from build123d import *

# Parameters (mm, degrees)
BOSS_EXTRUDE1_DEPTH             = 85
BOSS_EXTRUDE1_DEPTH_BACK        = 85
BOSS_EXTRUDE2_START             = -85
SKETCH1_4_W                     = 45
SKETCH1_4_H                     = 163
BOSS_EXTRUDE2_DEPTH             = 3
BOSS_EXTRUDE3_START             = 85
SKETCH1_5_W                     = 45
SKETCH1_5_H                     = 163
BOSS_EXTRUDE3_DEPTH             = 3
BOSS_EXTRUDE4_REACH             = 192.625
BOSS_EXTRUDE4_DIRECTION_2_REACH = 192.625
SKETCH5_W                       = 10
SKETCH5_H                       = 3
BOSS_EXTRUDE7_DEPTH             = 5
BOSS_EXTRUDE8_DEPTH             = 88
BOSS_EXTRUDE8_DEPTH_BACK        = 88
CHAMFER1_SIZE                   = 5


with BuildPart() as part:
    # Sketch1 → Boss-Extrude1 (new, two sides: drawn at the far end of the back side and taken through both)
    with BuildSketch(Plane(origin=(0, 0, 0), x_dir=(0, 0, -1), z_dir=(1, 0, 0)).offset(-BOSS_EXTRUDE1_DEPTH_BACK)):
        Polygon((-45, -3), (-45, 0), (0, 0), (0, 163), (3, 163), (3, -3), align=None)
    extrude(amount=BOSS_EXTRUDE1_DEPTH + BOSS_EXTRUDE1_DEPTH_BACK)

    # Sketch1<4> → Boss-Extrude2 (add)
    with BuildSketch(Plane(origin=(0, 0, 0), x_dir=(0, 0, -1), z_dir=(1, 0, 0)).offset(BOSS_EXTRUDE2_START)):
        with Locations((-22.5, 81.5)):
            Rectangle(SKETCH1_4_W, SKETCH1_4_H)
        Polygon((-45, -3), (-45, 0), (0, 0), (0, 163), (3, 163), (3, -3), align=None)
    extrude(amount=-BOSS_EXTRUDE2_DEPTH)

    # Sketch1<5> → Boss-Extrude3 (add)
    with BuildSketch(Plane(origin=(0, 0, 0), x_dir=(0, 0, -1), z_dir=(1, 0, 0)).offset(BOSS_EXTRUDE3_START)):
        Polygon((-45, -3), (-45, 0), (0, 0), (0, 163), (3, 163), (3, -3), align=None)
        with Locations((-22.5, 81.5)):
            Rectangle(SKETCH1_5_W, SKETCH1_5_H)
    extrude(amount=BOSS_EXTRUDE3_DEPTH)

    # Sketch2 → Boss-Extrude4 (add, up to next)
    with BuildSketch(Plane(origin=(0, 0, 0), x_dir=(0, 0, -1), z_dir=(1, 0, 0)), mode=Mode.PRIVATE) as boss_extrude4_sk1:
        Polygon((-10, 160), (-10, 150), (0, 140), (0, 160), align=None)
    boss_extrude4_tool1 = extrude(boss_extrude4_sk1.sketch, amount=BOSS_EXTRUDE4_REACH, mode=Mode.PRIVATE) - part.part
    add(boss_extrude4_tool1.solids().sort_by_distance((0, 152.222222, 4.444444))[0])

    # Sketch2 → Boss-Extrude4 direction 2 (add, up to next)
    with BuildSketch(Plane(origin=(0, 0, 0), x_dir=(0, 0, -1), z_dir=(1, 0, 0)), mode=Mode.PRIVATE) as boss_extrude4_direction_2_sk1:
        Polygon((-10, 160), (-10, 150), (0, 140), (0, 160), align=None)
    boss_extrude4_direction_2_tool1 = extrude(boss_extrude4_direction_2_sk1.sketch, amount=-BOSS_EXTRUDE4_DIRECTION_2_REACH, mode=Mode.PRIVATE) - part.part
    add(boss_extrude4_direction_2_tool1.solids().sort_by_distance((0, 152.222222, 4.444444))[0])

    # Sketch5 → Boss-Extrude7 (add)
    with BuildSketch(Plane(origin=(0, 0, 0), x_dir=(1, 0, 0), z_dir=(0, 1, 0))):
        with Locations((-45, -38.2)):
            Rectangle(SKETCH5_W, SKETCH5_H)
        with Locations((45, -38.2)):
            Rectangle(SKETCH5_W, SKETCH5_H)
        with Locations((0, -38.2)):
            Rectangle(SKETCH5_W, SKETCH5_H)
    extrude(amount=BOSS_EXTRUDE7_DEPTH)

    # Sketch4 → Boss-Extrude8 (add, two sides: drawn at the far end of the back side and taken through both)
    with BuildSketch(Plane(origin=(0, 0, 0), x_dir=(0, 0, -1), z_dir=(1, 0, 0)).offset(-BOSS_EXTRUDE8_DEPTH_BACK)):
        Polygon((-45, -3), (-48.742573267, -3), (-48.742573267, 0), (-45, 4), (-45, 0), align=None)
    extrude(amount=BOSS_EXTRUDE8_DEPTH + BOSS_EXTRUDE8_DEPTH_BACK)

    # Chamfer1
    chamfer1_edges = [part.edges().sort_by_distance(p)[0] for p in [
        (0, 0, 36.7),
        (45, 0, 36.7),
        (-45, 0, 36.7),
    ]]
    chamfer(chamfer1_edges, length=CHAMFER1_SIZE - 0.0001)  # a hair under: the kernel refuses the full size


solid = part.part
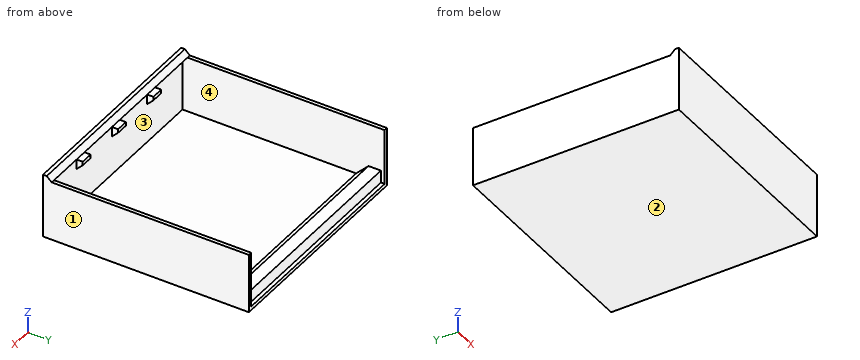
For this review, take the finished solid that the model builds, in its own axes (mm). Face numbers are marked on the shaded views. Round coordinates to 2 decimals unless told otherwise and drop trailing zeros. Order: outer loops, then holes, each group sorted by start corner. A loop starts at its lowest first (then second) coordinate and runs counter-clockwise, first axis right, second up. Notation, with made-up numbers: (3.25, 55.25) -> (21.25, 55.25) arc R21 ccw to (21.25, 93.25) -> close; hole circle Ø4 at (43.25, -5.75). An arc over 180 degrees is marked (long way). Put each result on its own line as item: value.
Q1. Add section A-A on z = 6. Write out the cut boundary in (x, y).
Check result:
outline: (-88, -3) -> (88, -3) -> (88, 163) -> (85, 163) -> (85, 160) -> (-85, 160) -> (-85, 163) -> (-88, 163) -> close; hole (-85, 0) -> (85, 0) -> (85, 146) -> (-85, 146) -> close
Q2. Mouldability with a two-part tool opening along X and no side actions: class the marked faces 1, 2, 3 and 4 as pulls with the +X half, pulls with the -X half, needs draft (parallel to the pull), parting line crosses it, or undercut.
Check result:
face 1: pulls with the +X half
face 2: needs draft
face 3: undercut
face 4: undercut
Q3. Add section C-C on y = 17.5. Write out the cut boundary in (x, z), plus the area to 3 significant figures.
Check result:
outline: (-88, -3) -> (88, -3) -> (88, 45) -> (85, 45) -> (85, 0) -> (-85, 0) -> (-85, 45) -> (-88, 45) -> close
area: 798 mm2
Q4. Add section D-D on z = 22. Write out the cut boundary in (x, y).
Check result:
outline: (-88, -3) -> (88, -3) -> (88, 163) -> (85, 163) -> (85, 0) -> (-85, 0) -> (-85, 163) -> (-88, 163) -> close
Q5. For probe 1 along X at (y, z) = (149, 22); probe 2 along Y at (x, z) = (-37, 27.5), list the stretches that pass through material, from the lowest coordinate up. Write a range as [from, to].
Check result:
probe 1: [-88, -85], [85, 88]
probe 2: [-3, 0]
Q6. Insertion check: pin 1 Ø3.5 at (x, z) = (42.5, 37.5) entering from +Y; pin 2 Ø4 at (x, y) = (-2, 1.5) entering from +Z; pin 3 Ø3.5 at (x, y) = (-86, 113.5) entering from +Z; pin 4 Ø1.5 at (x, y) = (-13.5, 136) entering from +Z. Each pin has a flat end and moves straight along its axis. Give the tip position at first contact, or say it passes through.
Check result:
pin 1: y = 5
pin 2: z = 48.74
pin 3: z = 45
pin 4: z = 0
